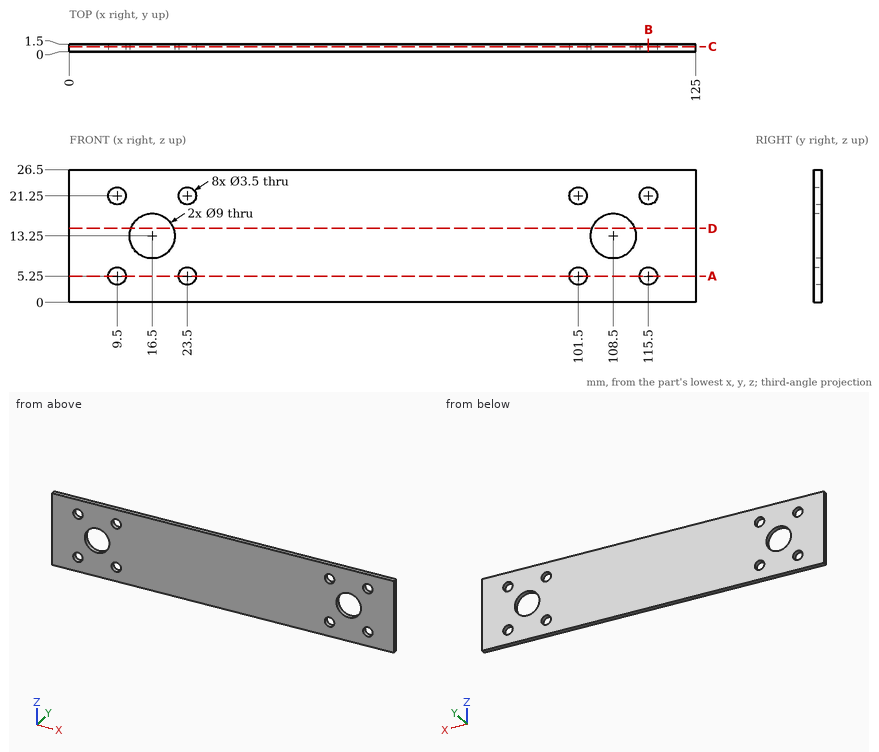
Part print with two shaded views. Sizes in mm from the minimum x, y, z corner. Round coordinates to 2 decimals unless told otherwise and drop trailing zeros. Order: outer loops, then holes, each group sorted by start corner. A loop starts at its lowest first (then second) coordinate and runs counter-clockwise, first axis right, second up. Notation, with made-up numbers: M -32.75,31 L -25.75,31 A26 cw -25.75,66 Z; hole C -4,-13 d9. An arc over 180 degrees is marked long. Put each result on its own line as item: value. Start each with the question number.
1. Slice it at B-B on x = 115.5. List the corners of the cut face in (y, z), then the cut area to 4 significant figures.
2. Slice it at D-D on z = 14.75. List the corners of the cut face in (x, y), then the cut area to 3 significant figures.
3. Slice it at A-A on z = 5.25. List the corners of the cut face in (x, y), then the cut area to 4 significant figures.
4. Drop a flat-ended pin along its axis: pin 1 (2 mm diameter, centred on x = 23.5, z = 5.25, fed in from +Y). Give the stop position or say it passes through.
5. Drill centre lines: probe 1 along X at (y, z) = (1, 13.25); probe 2 along Z at (x, y) = (9.5, 0.8); probe 3 along X at (y, z) = (0.85, 21.25). Where is each one in solid material? Low to high. Write a range as [from, to].
6. Slice it at C-C on y = 1. State how many separate pieces and enclosed holes the cut face has, then the cut area to 3 significant figures.
Findings:
1. outline: M 0,0 L 1.5,0 L 1.5,3.5 L 0,3.5 Z; M 0,7 L 1.5,7 L 1.5,19.5 L 0,19.5 Z; M 0,23 L 1.5,23 L 1.5,26.5 L 0,26.5 Z
1. area: 29.25 mm2
2. outline: M 0,0 L 12.26,0 L 12.26,1.5 L 0,1.5 Z; M 20.74,0 L 104.26,0 L 104.26,1.5 L 20.74,1.5 Z; M 112.74,0 L 125,0 L 125,1.5 L 112.74,1.5 Z
2. area: 162 mm2
3. outline: M 0,0 L 7.75,0 L 7.75,1.5 L 0,1.5 Z; M 11.25,0 L 21.75,0 L 21.75,1.5 L 11.25,1.5 Z; M 25.25,0 L 99.75,0 L 99.75,1.5 L 25.25,1.5 Z; M 103.25,0 L 113.75,0 L 113.75,1.5 L 103.25,1.5 Z; M 117.25,0 L 125,0 L 125,1.5 L 117.25,1.5 Z
3. area: 166.5 mm2
4. pin 1: through
5. probe 1: [0, 12], [21, 104], [113, 125]
5. probe 2: [0, 3.5], [7, 19.5], [23, 26.5]
5. probe 3: [0, 7.75], [11.25, 21.75], [25.25, 99.75], [103.25, 113.75], [117.25, 125]
6. separate pieces: 1
6. enclosed holes: 10
6. area: 3,110 mm2
